Part model, mm, in its own coordinate system. Face numbers are marked on the shaded views. A direction names the side the tool comes from. Coordinates: 2 decimals unless noted, no trailing zeros. Order: outer loops, then holes, each group sorted by start corner. A loop starts at its lowest first (then second) coordinate and runs counter-clockwise, first axis right, second up.
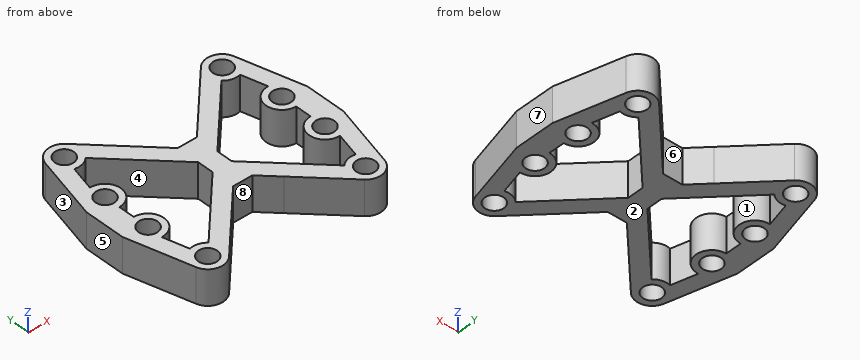
```python
from build123d import *

# Parameters (mm, degrees)
BOSS_EXTRUDE1_DEPTH = 6.985
SKETCH3_R           = 1.905
CUT_EXTRUDE1_DEPTH  = 31.093908852


with BuildPart() as part:
    # Sketch1 → Boss-Extrude1 (new body)
    with BuildSketch(Plane.XY):
        with BuildLine():
            Line((-5.23875, -9.525), (-13.603110789, -18.092914429))
            ThreePointArc((-13.603110789, -18.092914429), (-16.692674217, -18.942903824), (-18.949374194, -16.66799957))
            Line((-18.949374194, -16.66799957), (-22.225, -3.96875))
            Line((-22.225, -3.96875), (-22.225, 3.96875))
            Line((-22.225, 3.96875), (-18.949374194, 16.66799957))
            ThreePointArc((-18.949374194, 16.66799957), (-16.692674217, 18.942903824), (-13.603110789, 18.092914429))
            Line((-13.603110789, 18.092914429), (-5.23875, 9.525))
            Line((-5.23875, 9.525), (5.23875, 9.525))
            Line((5.23875, 9.525), (13.603110789, 18.092914429))
            ThreePointArc((13.603110789, 18.092914429), (16.692674217, 18.942903824), (18.949374194, 16.66799957))
            Line((18.949374194, 16.66799957), (22.225, 3.96875))
            Line((22.225, 3.96875), (22.225, -3.96875))
            Line((22.225, -3.96875), (18.949374194, -16.66799957))
            ThreePointArc((18.949374194, -16.66799957), (16.692674217, -18.942903824), (13.603110789, -18.092914429))
            Line((13.603110789, -18.092914429), (5.23875, -9.525))
            Line((5.23875, -9.525), (-5.23875, -9.525))
        make_face()
    extrude(amount=BOSS_EXTRUDE1_DEPTH)

    # Sketch3 → Cut-Extrude1 (cut, through all)
    with BuildSketch(Plane.XY.offset(6.985)):
        with Locations((-15.875, 15.875)):
            Circle(SKETCH3_R)
        with Locations((-17.78, 4.7625)):
            Circle(SKETCH3_R)
        with Locations(Location((17.78, 4.7625, 0), (0, 0, 180))):
            Circle(SKETCH3_R)
        with Locations((17.78, -4.7625)):
            Circle(SKETCH3_R)
        with Locations(Location((-17.78, -4.7625, 0), (0, 0, 180))):
            Circle(SKETCH3_R)
        with Locations(Location((15.875, 15.875, 0), (0, 0, 180))):
            Circle(SKETCH3_R)
        with Locations((15.875, -15.875)):
            Circle(SKETCH3_R)
        with Locations(Location((-15.875, -15.875, 0), (0, 0, 180))):
            Circle(SKETCH3_R)
        Polygon((-1.926937637, 6.132591943), (1.926937637, 6.132591943), (5.23875, 9.525), (-5.23875, 9.525), align=None)
        with BuildLine():
            Line((-17.922387107, 7.9375), (-16.66799957, 12.800625806))
            ThreePointArc((-16.66799957, 12.800625806), (-15.057325783, 12.807096176), (-13.657085571, 13.603110789))
            Line((-13.657085571, 13.603110789), (-1.926937637, 1.5875))
            Line((-1.926937637, 1.5875), (-1.926937637, -1.5875))
            Line((-1.926937637, -1.5875), (-13.657085571, -13.603110789))
            ThreePointArc((-13.657085571, -13.603110789), (-15.057325783, -12.807096176), (-16.66799957, -12.800625806))
            Line((-16.66799957, -12.800625806), (-17.922387107, -7.9375))
            Line((-17.922387107, -7.9375), (-17.78, -7.9375))
            ThreePointArc((-17.78, -7.9375), (-14.605, -4.7625), (-17.78, -1.5875))
            Line((-17.78, -1.5875), (-17.78, 1.5875))
            ThreePointArc((-17.78, 1.5875), (-14.605, 4.7625), (-17.78, 7.9375))
            Line((-17.78, 7.9375), (-17.922387107, 7.9375))
        make_face()
        with BuildLine():
            Line((17.922387107, -7.9375), (16.66799957, -12.800625806))
            ThreePointArc((16.66799957, -12.800625806), (15.057325783, -12.807096176), (13.657085571, -13.603110789))
            Line((13.657085571, -13.603110789), (1.926937637, -1.5875))
            Line((1.926937637, -1.5875), (1.926937637, 1.5875))
            Line((1.926937637, 1.5875), (13.657085571, 13.603110789))
            ThreePointArc((13.657085571, 13.603110789), (15.057325783, 12.807096176), (16.66799957, 12.800625806))
            Line((16.66799957, 12.800625806), (17.922387107, 7.9375))
            Line((17.922387107, 7.9375), (17.78, 7.9375))
            ThreePointArc((17.78, 7.9375), (14.605, 4.7625), (17.78, 1.5875))
            Line((17.78, 1.5875), (17.78, -1.5875))
            ThreePointArc((17.78, -1.5875), (14.605, -4.7625), (17.78, -7.9375))
            Line((17.78, -7.9375), (17.922387107, -7.9375))
        make_face()
        Polygon((-5.23875, -9.525), (5.23875, -9.525), (1.926937637, -6.132591943), (-1.926937637, -6.132591943), align=None)
    extrude(amount=-CUT_EXTRUDE1_DEPTH, mode=Mode.SUBTRACT)


solid = part.part
```
(1) Tool access for the marked faces 4, 5, 6, 7 and 8: list every direction of +Z, -Z, +X, -X, +Y, -Y with a clear straight run to the whole face (end or side of a thin tool).
(2) Pull direction X, two halves, no side cores. Call the marked faces 1, 2 and 3: +X half, -X half, draft (parallel to the pull), parting line (faces both ways), or undercut.
(3) Slice it at C-C, the plane z = 1.75. State how many separate pieces and enclosed holes the cut face has, then the cut area to 3 significant figures.
(4) Slice it at B-B, the plane x = -4. Give the cut face in (y, z) (3 decimals), then the cut area to 3 significant figures.
(5) Slice it at A-A, the plane y = -0.5. Give the cut face in (x, z) (3 decimals).
(6) Drop flat-ended pins along their axis: pin 1 (1.5 mm diameter, centred on x = -2.5, z = 4, fed in from -Y); pin 2 (4 mm diameter, centred on x = -1, z = 2.5, fed in from -Y); pin 3 (1.5 mm diameter, centred on x = -0.5, z = 6, fed in from +Y). Give the stop position or say it passes through.
(7) Probe line 1 (X direction, y = 12, z = 5.5); line 2 (X direction, y = 5.5, z = 2.75); line 3 (X direction, y = -5, z = 2.25). List the from-to ranges inside material, lowest first.
Here are the results:
1. face 4: +Z, -Z
1. face 5: +Z, -Z, -X, +Y, -Y
1. face 6: +Z, -Z, +Y
1. face 7: +Z, -Z, +X, +Y, -Y
1. face 8: +Z, -Z, -Y
2. face 1: undercut
2. face 2: draft
2. face 3: -X half
3. separate pieces: 1
3. enclosed holes: 10
3. area: 558 mm2
4. outline: (-8.256, 0) - (-3.711, 0) - (-3.711, 6.985) - (-8.256, 6.985) - close; (3.711, 0) - (8.256, 0) - (8.256, 6.985) - (3.711, 6.985) - close
4. area: 63.5 mm2
5. outline: (-22.225, 0) - (-17.78, 0) - (-17.78, 6.985) - (-22.225, 6.985) - close; (-1.927, 0) - (1.927, 0) - (1.927, 6.985) - (-1.927, 6.985) - close; (17.78, 0) - (22.225, 0) - (22.225, 6.985) - (17.78, 6.985) - close
6. pin 1: stops at y = -7.49
6. pin 2: stops at y = -7.23
6. pin 3: stops at y = 6.13
7. line 1: x = -20.15 to -16.87, -12.09 to -7.65, 7.65 to 12.09, 16.87 to 20.15
7. line 2: x = -21.83 to -19.54, -16.02 to -14.69, -5.75 to 5.75, 14.69 to 16.02, 19.54 to 21.83
7. line 3: x = -21.96 to -19.67, -15.89 to -14.61, -5.26 to 5.26, 14.61 to 15.89, 19.67 to 21.96
